Can you work these out from the model? Positions are in its coordinate system, mm. A direction names the side the tool comes from. Give positions to 0.01 mm unless a question says otherwise; leave off trailing zeros. Answer as a JSON object with one key per item and string values.
```python
from build123d import *

# Parameters (mm, degrees)
SKETCH2_W                = 50
SKETCH2_H                = 50
FILLET2_R                = 10
SKETCH3_R                = 60
BOSS_EXTRUDE2_DEPTH      = 20
BOSS_EXTRUDE2_DEPTH_BACK = 20
CUT_EXTRUDE1_DEPTH       = 46
CIRPATTERN1_COUNT        = 10


with BuildPart() as part:
    # Sketch2 → Revolve1 (revolve)
    with BuildSketch(Plane.XY):
        with Locations((-75, 0)):
            Rectangle(SKETCH2_W, SKETCH2_H)
    revolve(axis=Axis((0, 0, 0), (0, 1, 0)))

    # Fillet2
    fillet2_edges = [part.edges().sort_by_distance(p)[0] for p in [
        (50, 25, 0),
        (100, 25, 0),
        (100, -25, 0),
        (50, -25, 0),
    ]]
    fillet(fillet2_edges, radius=FILLET2_R)

    # Sketch3 → Boss-Extrude2 (add, two sides)
    with BuildSketch(Plane(origin=(0, 0, 0), x_dir=(1, 0, 0), z_dir=(0, 1, 0))) as boss_extrude2_sk:
        Circle(SKETCH3_R)
    extrude(amount=BOSS_EXTRUDE2_DEPTH)
    extrude(boss_extrude2_sk.sketch, amount=-BOSS_EXTRUDE2_DEPTH_BACK)

    # Sketch4 → Cut-Extrude1 (cut, through all)
    with BuildSketch(Plane.XZ.offset(20)):
        with BuildLine():
            ThreePointArc((-1.631577403, 12.393060767), (0, 12.5), (1.631577403, 12.393060767))
            Line((1.631577403, 12.393060767), (6.048550589, 45.943303012))
            ThreePointArc((6.048550589, 45.943303012), (0, 46.339745962), (-6.048550589, 45.943303012))
            Line((-6.048550589, 45.943303012), (-1.631577403, 12.393060767))
        make_face()
    cut_extrude1 = extrude(amount=-CUT_EXTRUDE1_DEPTH, mode=Mode.SUBTRACT)

    # CirPattern1: Cut-Extrude1 ×10 about axis
    cirpattern1_axis = Axis((0, 0, 0), (0, 1, 0))
    for i in range(1, CIRPATTERN1_COUNT):
        add(cut_extrude1.rotate(cirpattern1_axis, i * 360 / CIRPATTERN1_COUNT), mode=Mode.SUBTRACT)


solid = part.part
```
1) I'm going to push flat-ended pins straight in: P1, Ø8, axis at y = -10, z = -61.5, coming from the -X side; P2, Ø6, axis at x = 37, y = -17, coming from the -Z side; P3, Ø10, axis at x = -52, y = -6, coming from the -Z side. Where does each tip first touch, or does it pass through?
Check sheet entries:
{"P1": "x = -81.82", "P2": "z = -93.93", "P3": "z = -88.27"}
2) I need wall thicknesses on L1, parallel to Z at x = -11, y = 8; L2, parallel to Z at x = -31, y = -10.5; L3, parallel to X at y = 16.5, z = 12. Which ranges of each line are inside material? Lowest first, please.
Check sheet entries:
{"L1": "-99.39 to -20.26, -11.59 to 11.59, 20.26 to 99.39", "L2": "-95.07 to -34.44, -32.67 to -14.79, -5.75 to 5.75, 14.79 to 32.67, 34.44 to 95.07", "L3": "-99.16 to -44.76, -25.16 to -11.39, -6.52 to 6.52, 11.39 to 25.16, 44.76 to 99.16"}
3) If we mould it in two halves opening along Z, with no side actions, what happens to faces 1 (the cylindrical face through (-95.38, 0.21, 30.04)), 2 (the flat face through (20.09, -0.28, 21.17)), 3 (the flat face through (-59, -25, -19))? For each: released by +Z, released by -Z, zero draft, split by the parting line, or undercut.
Check sheet entries:
{"face 1": "split by the parting line", "face 2": "undercut", "face 3": "zero draft"}
4) Imagine slicing it at A-A on y = -7. Give the number of separate pieces and of enclosed holes in the cut face, and give its area (3 significant figures).
Check sheet entries:
{"separate pieces": "1", "enclosed holes": "10", "area": "28,800 mm2"}
5) Which directions (+Z, -Z, +X, -X, +Y, -Y) give clear straight access to the entire face, cutting with the end or side of a thin tool? Please do faces 4 (the flat face through (-1, -20, -1)), 5 (the cylindrical face through (-0.08, -0.28, -46.34)).
Check sheet entries:
{"face 4": "-Y", "face 5": "+Y, -Y"}
